```python
from build123d import *

# Parameters (mm, degrees)
SKETCH_1_R          = 3.5
EXTRUDE_1_DEPTH     = 60
SKETCH_2_R          = 6.25
CUT_EXTRUDE_1_DEPTH = 20
CUT_EXTRUDE_START   = -20
SKETCH_3_R          = 6.25
CUT_EXTRUDE_2_DEPTH = 20
SKETCH_4_R          = 3.5
CUT_EXTRUDE_3_DEPTH = 4
SKETCH_5_R          = 3.5
CUT_EXTRUDE_4_DEPTH = 4
SKETCH_6_R          = 1.75
CUT_EXTRUDE_5_DEPTH = 14
SKETCH_7_R          = 1.75
CUT_EXTRUDE_6_DEPTH = 10
CUT_EXTRUDE_START_2 = -10
SKETCH_8_R          = 1.75
CUT_EXTRUDE_7_DEPTH = 10


with BuildPart() as part:
    # 草图1 → 凸台-拉伸1 (new body)
    with BuildSketch(Plane.XY):
        with BuildLine():
            Line((38.795098039, 43.765686275), (1.795098039, 43.765686275))
            ThreePointArc((1.795098039, 43.765686275), (0.734437867, 43.326346446), (0.295098039, 42.265686275))
            Line((0.295098039, 42.265686275), (0.295098039, 30.265686275))
            ThreePointArc((0.295098039, 30.265686275), (0.734437867, 31.326346446), (1.795098039, 31.765686275))
            Line((1.795098039, 31.765686275), (38.795098039, 31.765686275))
            ThreePointArc((38.795098039, 31.765686275), (39.855758211, 31.326346446), (40.295098039, 30.265686275))
            Line((40.295098039, 30.265686275), (40.295098039, 42.265686275))
            ThreePointArc((40.295098039, 42.265686275), (39.855758211, 43.326346446), (38.795098039, 43.765686275))
        make_face()
        with Locations((30.295098039, 36.405686275)):
            Circle(SKETCH_1_R, mode=Mode.SUBTRACT)
        with Locations((10.295098039, 36.405686275)):
            Circle(SKETCH_1_R, mode=Mode.SUBTRACT)
    extrude(amount=EXTRUDE_1_DEPTH)

    # 草图2 → 切除-拉伸1 (cut)
    with BuildSketch(Plane.XY.offset(60)):
        with Locations((10.295098039, 36.405686275)):
            Circle(SKETCH_2_R)
        with Locations((30.295098039, 36.405686275)):
            Circle(SKETCH_2_R)
    extrude(amount=-CUT_EXTRUDE_1_DEPTH, mode=Mode.SUBTRACT)

    # 草图3 → 切除-拉伸2 (cut)
    with BuildSketch(Plane(origin=(0, 0, 0), x_dir=(-1, 0, 0), z_dir=(0, 0, -1)).offset(CUT_EXTRUDE_START)):
        with Locations((-10.295098039, 36.405686275)):
            Circle(SKETCH_3_R)
        with Locations((-30.295098039, 36.405686275)):
            Circle(SKETCH_3_R)
    extrude(amount=CUT_EXTRUDE_2_DEPTH, mode=Mode.SUBTRACT)

    # 草图4 → 切除-拉伸3 (cut)
    with BuildSketch(Plane(origin=(0, 43.765686275, 0), x_dir=(1, 0, 0), z_dir=(0, 1, 0))):
        with Locations(Location((20.295098039, -30, 0), (0, 0, 270))):
            Circle(SKETCH_4_R)
    extrude(amount=-CUT_EXTRUDE_3_DEPTH, mode=Mode.SUBTRACT)

    # 草图5 → 切除-拉伸4 (cut)
    with BuildSketch(Plane(origin=(0, 43.765686275, 0), x_dir=(1, 0, 0), z_dir=(0, 1, 0))):
        with Locations(Location((20.295098039, -15, 0), (0, 0, 270))):
            Circle(SKETCH_5_R)
        with Locations(Location((20.295098039, -45, 0), (0, 0, 270))):
            Circle(SKETCH_5_R)
    extrude(amount=-CUT_EXTRUDE_4_DEPTH, mode=Mode.SUBTRACT)

    # 草图6 → 切除-拉伸5 (cut)
    with BuildSketch(Plane(origin=(0, 39.765686275, 0), x_dir=(1, 0, 0), z_dir=(0, 1, 0))):
        with Locations(Location((20.295098039, -30, 0), (0, 0, 270))):
            Circle(SKETCH_6_R)
        with Locations(Location((20.295098039, -15, 0), (0, 0, 270))):
            Circle(SKETCH_6_R)
        with Locations(Location((20.295098039, -45, 0), (0, 0, 270))):
            Circle(SKETCH_6_R)
    extrude(amount=-CUT_EXTRUDE_5_DEPTH, mode=Mode.SUBTRACT)

    # 草图7 → 切除-拉伸6 (cut)
    with BuildSketch(Plane.XY.offset(60)):
        with Locations((20.295098039, 36.405686275)):
            Circle(SKETCH_7_R)
    extrude(amount=-CUT_EXTRUDE_6_DEPTH, mode=Mode.SUBTRACT)

    # 草图8 → 切除-拉伸7 (cut)
    with BuildSketch(Plane(origin=(0, 0, 0), x_dir=(-1, 0, 0), z_dir=(0, 0, -1)).offset(CUT_EXTRUDE_START_2)):
        with Locations(Location((-20.295098039, 36.405686275, 0), (0, 0, 180))):
            Circle(SKETCH_8_R)
    extrude(amount=CUT_EXTRUDE_7_DEPTH, mode=Mode.SUBTRACT)


solid = part.part
```
Work out the finished part from the listing and answer in its coordinate system (mm). A direction names the side the tool comes from. Coordinates: 2 decimals unless noted, no trailing zeros. Loops run counter-clockwise (first coordinate to the right, second up) from the corner with the lowest first, then second, coordinate; pieces in that order, holes last. Notation, with made-up numbers: M 15,-31.5 L 21,-31.5 A15 ccw 21,-27.5 Z; hole C -30,33 d9. An arc over 180 degrees is marked long. Use CSV: the item, a comma, the result in double quotes. Start each with the question number.
(1) For a pull along Y with two mould halves and no side action, classify faces 1 (the face through (20, 39.766, 43)), 2 (the face through (20, 39, 60)), 3 (the face through (0.72, 31.31, 29.58)), 4 (the face through (20.07, 38.14, 55.07)) as +Y half, -Y half, draft (parallel to the pull), parting line (faces both ways), or undercut.
(2) Find section A-A, the plane y = 33.5. State how many separate pieces and enclosed holes the cut face has, then the cut area to 3 significant figures.
(3) Given pin 1 Ø4.5 at (x, z) = (20.3, 30) entering from -Y; pin 2 Ø9 at (x, z) = (20.3, 45) entering from +Y; pin 3 Ø2 at (x, z) = (20.5, 13.5) entering from +Y; pin 4 Ø5 at (x, y) = (13.5, 37) entering from -Z, each flat-ended and moving along its own axis, determine where each tip first touches the part or whether it passes through.
(4) Find section B-B, the plane z = 15. Give the vertices of the cut face in (x, y).
(5) For faces 5 (the face through (13.53, 35.07, 29.86)), 6 (the face through (24, 31.766, 30)), 7 (the face through (18.95, 41.79, 33.23)), 8 (the face through (12, 40, 40)), 9 (the face through (29, 40, 20)), determine the directions among +Z, -Z, +X, -X, +Y, -Y from which every point of the face is accessible in a straight line to the end or side of a thin tool.
(6) Find section C-C, the plane x = 9. Give the vertices of the cut face in (y, z).
(7) Find section D-D, the plane z = 29. Give the vertices of the cut face in (x, y), then the cut area to 3 significant figures.
(8) Consider line 1 (Z direction, x = 21.5, y = 41.5); line 2 (X direction, y = 35.75, z = 36.5); line 3 (X direction, y = 35, z = 55.5). Determine where each line is inside the solid, lowest interval first.
Recorded:
1,face 1,"+Y half"
1,face 2,"draft"
1,face 3,"-Y half"
1,face 4,"undercut"
2,separate pieces,"3"
2,enclosed holes,"3"
2,area,"1,330 mm^2"
3,pin 1,"stops at y = 31.77"
3,pin 2,"stops at y = 43.77"
3,pin 3,"stops at y = 39.77"
3,pin 4,"stops at z = 20"
4,outline,"M 0.3,30.27 A1.5 cw 1.8,31.77 L 6.11,31.77 A6.25 cw long 14.48,31.77 L 18.55,31.77 L 18.55,39.77 L 16.8,39.77 L 16.8,43.77 L 1.8,43.77 A1.5 ccw 0.3,42.27 Z; M 22.05,31.77 L 26.11,31.77 A6.25 cw long 34.48,31.77 L 38.8,31.77 A1.5 cw 40.3,30.27 L 40.3,42.27 A1.5 ccw 38.8,43.77 L 23.8,43.77 L 23.8,39.77 L 22.05,39.77 Z"
5,face 5,"+Z, -Z"
5,face 6,"+Z, -Z, -Y"
5,face 7,"+Y"
5,face 8,"+Z"
5,face 9,"-Z"
6,outline,"M 31.77,20 L 33.15,20 L 33.15,40 L 31.77,40 Z; M 39.66,20 L 42.52,20 L 42.52,0 L 43.77,0 L 43.77,60 L 42.52,60 L 42.52,40 L 39.66,40 Z"
7,outline,"M 0.3,30.27 A1.5 cw 1.8,31.77 L 18.86,31.77 L 18.86,39.77 L 16.94,39.77 L 16.94,43.77 L 1.8,43.77 A1.5 ccw 0.3,42.27 Z; M 21.73,31.77 L 38.8,31.77 A1.5 cw 40.3,30.27 L 40.3,42.27 A1.5 ccw 38.8,43.77 L 23.65,43.77 L 23.65,39.77 L 21.73,39.77 Z; hole C 10.3,36.41 d7; hole C 30.3,36.41 d7"
7,area,"353 mm^2"
8,line 1,"z = 0 to 11.71, 18.29 to 26.71, 33.29 to 41.71, 48.29 to 60"
8,line 2,"x = 0.3 to 6.86, 13.73 to 26.86, 33.73 to 40.3"
8,line 3,"x = 0.3 to 4.21, 16.38 to 19.25, 21.34 to 24.21, 36.38 to 40.3"
